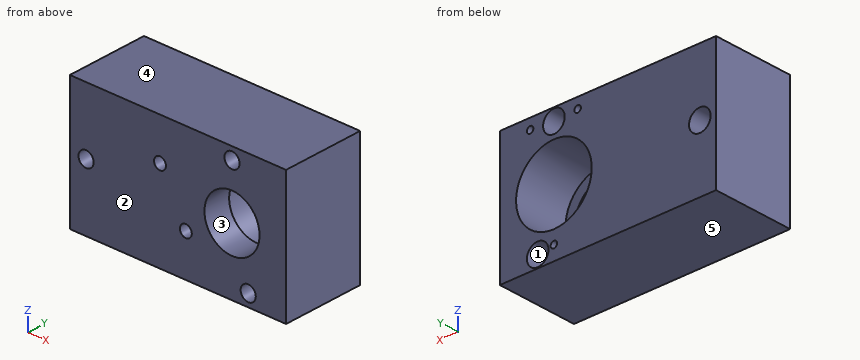
```python
from build123d import *

# Parameters (mm, degrees)
SKETCH_1_W          = 20
SKETCH_1_H          = 12
EXTRUDE_1_DEPTH     = 2.5
SKETCH_1_9_R        = 0.55
SKETCH_1_9_R_2      = 2.55
CUT_EXTRUDE_3_DEPTH = 2.5
EXTRUDE_START       = 2.5
SKETCH_1_10_W       = 20
SKETCH_1_10_H       = 12
SKETCH_1_10_R       = 3.5
EXTRUDE_2_DEPTH     = 5
SKETCH_2_R          = 0.7
CUT_EXTRUDE_4_DEPTH = 25.5
CUT_EXTRUDE_START   = -7.5
SKETCH_2_3_R        = 1
CUT_EXTRUDE_5_DEPTH = 5.5
SKETCH_2_6_R        = 0.3
CUT_EXTRUDE_6_DEPTH = 6


with BuildPart() as part:
    # 草图1 → 凸台-拉伸1 (new body)
    with BuildSketch(Plane(origin=(0, 0, 0), x_dir=(1, 0, 0), z_dir=(0, 1, 0))):
        with Locations((10, -6)):
            Rectangle(SKETCH_1_W, SKETCH_1_H)
    extrude(amount=EXTRUDE_1_DEPTH)

    # 草图1<9> → 切除-拉伸3 (cut)
    with BuildSketch(Plane(origin=(0, 0, 0), x_dir=(1, 0, 0), z_dir=(0, 1, 0))):
        with Locations(Location((8.340658618, -8.2, 0), (0, 0, 270))):
            Circle(SKETCH_1_9_R)
        with Locations(Location((10.72985855, -3.807765525, 0), (0, 0, 270))):
            Circle(SKETCH_1_9_R)
        with Locations(Location((15, -6, 0), (0, 0, 270))):
            Circle(SKETCH_1_9_R_2)
    extrude(amount=CUT_EXTRUDE_3_DEPTH, mode=Mode.SUBTRACT)

    # 草图1<10> → 凸台-拉伸2 (add)
    with BuildSketch(Plane(origin=(0, 0, 0), x_dir=(1, 0, 0), z_dir=(0, 1, 0)).offset(EXTRUDE_START)):
        with Locations((10, -6)):
            Rectangle(SKETCH_1_10_W, SKETCH_1_10_H)
        with Locations(Location((15, -6, 0), (0, 0, 90))):
            Circle(SKETCH_1_10_R, mode=Mode.SUBTRACT)
    extrude(amount=EXTRUDE_2_DEPTH)

    # 草图2 → 切除-拉伸4 (cut, through all)
    with BuildSketch(Plane.XZ):
        with Locations(Location((15, 10.9, 0), (0, 0, 270))):
            Circle(SKETCH_2_R)
        with Locations(Location((1.5, 6, 0), (0, 0, 270))):
            Circle(SKETCH_2_R)
        with Locations(Location((16.5, 1.1, 0), (0, 0, 270))):
            Circle(SKETCH_2_R)
    extrude(amount=-CUT_EXTRUDE_4_DEPTH, mode=Mode.SUBTRACT)

    # 草图2<3> → 切除-拉伸5 (cut)
    with BuildSketch(Plane.XZ.offset(CUT_EXTRUDE_START)):
        with Locations(Location((16.5, 1.1, 0), (0, 0, 90))):
            Circle(SKETCH_2_3_R)
        with Locations(Location((15, 10.9, 0), (0, 0, 90))):
            Circle(SKETCH_2_3_R)
        with Locations(Location((1.5, 6, 0), (0, 0, 90))):
            Circle(SKETCH_2_3_R)
    extrude(amount=CUT_EXTRUDE_5_DEPTH, mode=Mode.SUBTRACT)

    # 草图2<6> → 切除-拉伸6 (cut)
    with BuildSketch(Plane.XZ.offset(CUT_EXTRUDE_START)):
        with Locations(Location((12.8, 11.05, 0), (0, 0, 90))):
            Circle(SKETCH_2_6_R)
        with Locations(Location((17.2, 11.05, 0), (0, 0, 90))):
            Circle(SKETCH_2_6_R)
        with Locations(Location((15, 1.3, 0), (0, 0, 90))):
            Circle(SKETCH_2_6_R)
    extrude(amount=CUT_EXTRUDE_6_DEPTH, mode=Mode.SUBTRACT)


solid = part.part
```
The listing builds one solid part. Answer for the finished solid, in the listing's coordinates (mm). Face numbers are marked on the shaded views. A direction names the side the tool comes from. Coordinates: 2 decimals unless noted, no trailing zeros. Loops run counter-clockwise (first coordinate to the right, second up) from the corner with the lowest first, then second, coordinate; pieces in that order, holes last. Notation, with made-up numbers: (50.5, 80.25) -> (102.5, 80.25) arc R35 ccw to (102.5, 114.25) -> close; hole circle Ø6 at (72.25, 29). An arc over 180 degrees is marked (long way). Return JSON: item names as keys, results as strings. Group by question number.
(1) A cutting plane is placed at B-B on z = 11.05. Write down the section's boundary in (x, y), and give its area (3 significant figures).
(2) Find the intervals of material crossed by probe 1 along X at (y, z) = (5.5, 6); probe 2 along X at (y, z) = (0.6, 8.2); probe 3 along X at (y, z) = (1, 1.1), in increasing order. Write a range as from..to.
(3) A cutting plane is placed at D-D on z = 5.5. Write down the section's boundary in (x, y).
(4) Given pin 1 Ø2 at (y, z) = (5, 5.5) entering from -X; pin 2 Ø6.5 at (x, z) = (15, 6) entering from +Y; pin 3 Ø0.9 at (x, z) = (10.73, 3.81) entering from -Y, each flat-ended and moving along its own axis, determine where each tip first touches the part or whether it passes through.
(5) A cutting plane is placed at C-C on y = 4.75. Write down the section's boundary in (x, z).
(6) Determine the mould class of the marked faces 3, 4 and 5 for opening direction Z: released by +Z, released by -Z, zero draft, split by the parting line, or undercut.
(7) A cutting plane is placed at A-A on x = 1.5. Write down the section's boundary in (y, z).
(8) Which of the six approach directions +Z, -Z, +X, -X, +Y, -Y give full straight-line access (tool end or side, diameter ignored) to the marked faces 1 and 2?
The answers:
{
 "1": {"outline": "(0, 0) -> (14.32, 0) -> (14.32, 2) -> (14.01, 2) -> (14.01, 7.5) -> (13.1, 7.5) -> (13.1, 1.5) -> (12.5, 1.5) -> (12.5, 7.5) -> (0, 7.5) -> close; (15.68, 0) -> (20, 0) -> (20, 7.5) -> (17.5, 7.5) -> (17.5, 1.5) -> (16.9, 1.5) -> (16.9, 7.5) -> (15.99, 7.5) -> (15.99, 2) -> (15.68, 2) -> close", "area": "129 mm^2"},
 "2": {"probe 1": "x = 0..0.5, 2.5..11.5, 18.5..20", "probe 2": "x = 0..7.79, 8.89..13.71, 16.29..20", "probe 3": "x = 0..15.8, 17.2..20"},
 "3": {"outline": "(0, 0) -> (1.01, 0) -> (1.01, 2) -> (0.63, 2) -> (0.63, 7.5) -> (0, 7.5) -> close; (1.99, 0) -> (12.5, 0) -> (12.5, 2.5) -> (11.54, 2.5) -> (11.54, 7.5) -> (2.37, 7.5) -> (2.37, 2) -> (1.99, 2) -> close; (17.5, 0) -> (20, 0) -> (20, 7.5) -> (18.46, 7.5) -> (18.46, 2.5) -> (17.5, 2.5) -> close"},
 "4": {"pin 1": "stops at x = 0", "pin 2": "stops at y = 2.5", "pin 3": "stops at y = 2.5"},
 "5": {"outline": "(0, 0) -> (20, 0) -> (20, 12) -> (0, 12) -> close; hole circle Ø2 at (1.5, 6); hole circle Ø7 at (15, 6); hole circle Ø0.6 at (12.8, 11.05); hole circle Ø2 at (15, 10.9); hole circle Ø0.6 at (15, 1.3); hole circle Ø2 at (16.5, 1.1); hole circle Ø0.6 at (17.2, 11.05)"},
 "6": {"face 3": "undercut", "face 4": "released by +Z", "face 5": "released by -Z"},
 "7": {"outline": "(0, 0) -> (7.5, 0) -> (7.5, 5) -> (2, 5) -> (2, 5.3) -> (0, 5.3) -> close; (0, 6.7) -> (2, 6.7) -> (2, 7) -> (7.5, 7) -> (7.5, 12) -> (0, 12) -> close"},
 "8": {"face 1": "+Y", "face 2": "+Z, -Z, +X, -X, -Y"}
}
